Design review of the part shown in the three views and the two pictorial views. Dimensions are in mm from the part's minimum x, y and z. A direction names the side the tool comes from. Coordinates: 2 decimals unless noted, no trailing zeros. Loops run counter-clockwise (first coordinate to the right, second up) from the corner with the lowest first, then second, coordinate; pieces in that order, holes last.
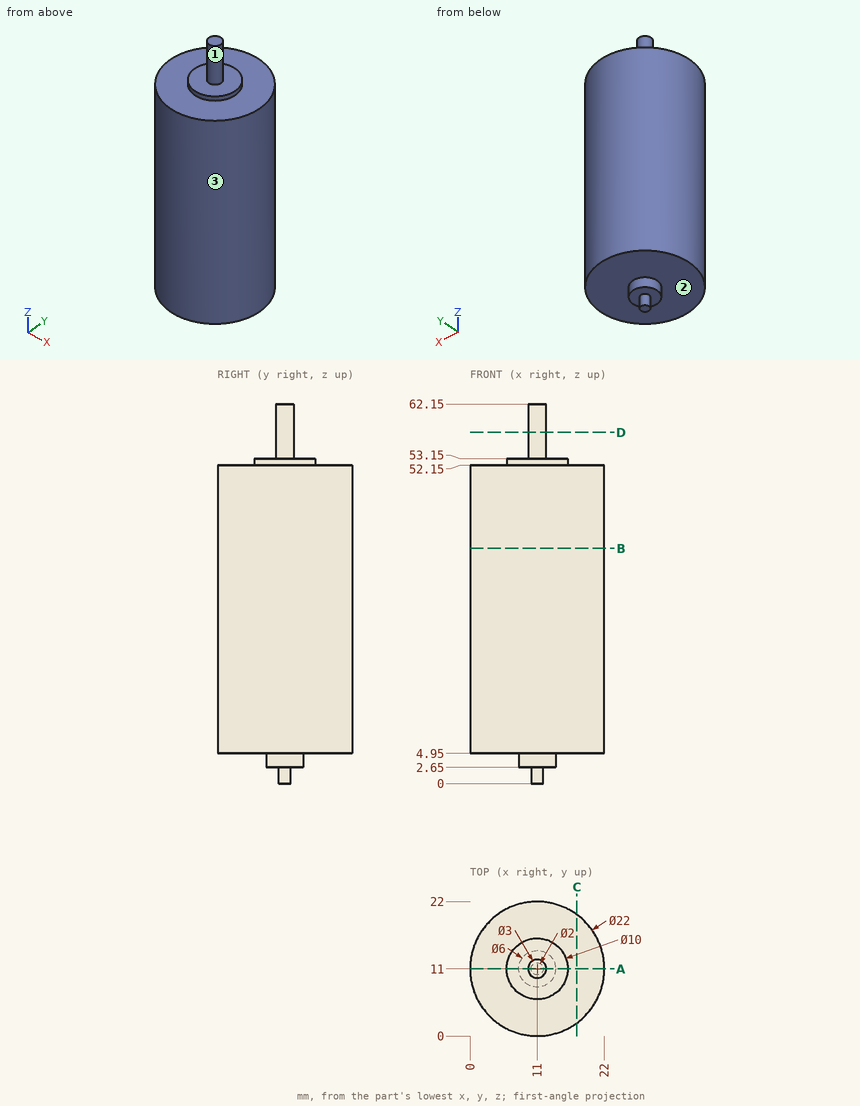
Q1. Consider section C-C (x = 17.5). State the section outline as (y, z) points.
Q2. Consider section A-A (y = 11). State the section outline as (x, z) points.
Q3. For pin 1 Ø6.5 at (x, y) = (10.5, 11) entering from -Z; pin 2 Ø6.5 at (x, y) = (7, 5.5) entering from +Z; pin 3 Ø1.5 at (x, z) = (13.5, 53) entering from +Y; pin 4 Ø5 at (y, z) = (3.5, 39) entering from -X, all flat-tipped, find the tip position at first contact; note any pin that passes through.
Q4. Machinability: for the marked faces 1, 2 and 3, which of the approach directions +Z, -Z, +X, -X, +Y, -Y give a long, thin tool a straight path to every point of the face, cutting with its end or side? Answer none if there is none.
Q5. Consider section B-B (z = 38.5). State the section outline as (x, y) points.
Q6. Consider section D-D (z = 57.5). State the section outline as (x, y) points.
Q7. Wall thickness on probe 1 along Z at (x, y) = (14.75, 18.25); probe 2 along X at (y, z) = (10.75, 46); probe 3 along Y at (x, z) = (15.5, 15.5): over which ranges is each line inside the solid? List them lowest first.
Model answer:
1. outline: (2.13, 4.95) - (19.87, 4.95) - (19.87, 52.15) - (2.13, 52.15) - close
2. outline: (0, 4.95) - (8, 4.95) - (8, 2.65) - (10, 2.65) - (10, 0) - (12, 0) - (12, 2.65) - (14, 2.65) - (14, 4.95) - (22, 4.95) - (22, 52.15) - (16, 52.15) - (16, 53.15) - (12.5, 53.15) - (12.5, 62.15) - (9.5, 62.15) - (9.5, 53.15) - (6, 53.15) - (6, 52.15) - (0, 52.15) - close
3. pin 1: stops at z = 0
3. pin 2: stops at z = 53.15
3. pin 3: stops at y = 15.68
3. pin 4: stops at x = 1.2
4. face 1: +Z
4. face 2: -Z
4. face 3: +Z, -Z
5. outline: circle Ø22 at (11, 11)
6. outline: circle Ø3 at (11, 11)
7. probe 1: z = 4.95 to 52.15
7. probe 2: x = 0 to 22
7. probe 3: y = 0.96 to 21.04
